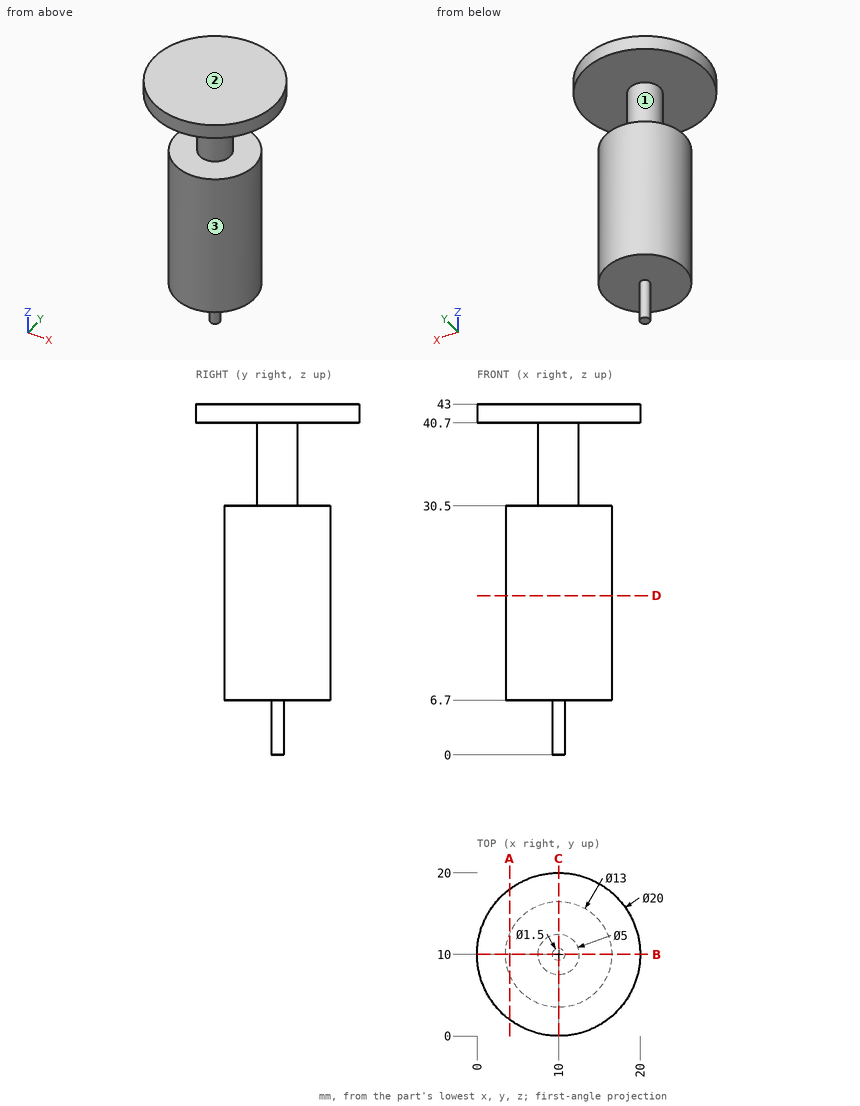
Input: dimensioned drawing with shaded views. Units: mm. Origin: part minimum x, y, z. A direction names the side the tool comes from. Give positions to 0.01 mm unless a question says otherwise; leave off trailing zeros. Loops run counter-clockwise (first coordinate to the right, second up) from the corner with the lowest first, then second, coordinate; pieces in that order, holes last. Notation, with made-up numbers: (31, 58.25) -> (55, 58.25) arc R23 cw to (55, 85.25) -> close; hole circle Ø9 at (-32, 10.5). An arc over 180 degrees is marked (long way). Use a Markdown table: item, result.
Q1. Ray query, probe 1 along Z at (x, y) = (5.5, 5.5); probe 2 along Z at (x, y) = (12, 17.75); probe 3 along X at (y, z) = (5.5, 41). Return the intervals inside material, ascending. Write a range as from..to.
Entries:
| item | result |
|---|---|
| probe 1 | z = 6.7..30.5, 40.7..43 |
| probe 2 | z = 40.7..43 |
| probe 3 | x = 1.07..18.93 |
Q2. Access query for the marked faces 1, 2 and 3. Directions: +Z, -Z, +X, -X, +Y, -Y. A direction counts if a zero-diameter tool reaches every point of the face in a straight line with its end or side. Return the directions, or none.
Entries:
| item | result |
|---|---|
| face 1 | none |
| face 2 | +Z, +X, -X, +Y, -Y |
| face 3 | -Z |
Q3. Section query B-B, the plane y = 10. Return the cut outline in (x, z).
Entries:
| item | result |
|---|---|
| outline | (0, 40.7) -> (7.5, 40.7) -> (7.5, 30.5) -> (3.5, 30.5) -> (3.5, 6.7) -> (9.25, 6.7) -> (9.25, 0) -> (10.75, 0) -> (10.75, 6.7) -> (16.5, 6.7) -> (16.5, 30.5) -> (12.5, 30.5) -> (12.5, 40.7) -> (20, 40.7) -> (20, 43) -> (0, 43) -> close |
Q4. Section query D-D, the plane z = 19.5. Return the cut outline in (x, y).
Entries:
| item | result |
|---|---|
| outline | circle Ø13 at (10, 10) |
Q5. Section query A-A, the plane x = 4. Return the cut outline in (y, z), plus the area to 3 significant figures.
Entries:
| item | result |
|---|---|
| outline | (2, 40.7) -> (18, 40.7) -> (18, 43) -> (2, 43) -> close; (7.5, 6.7) -> (12.5, 6.7) -> (12.5, 30.5) -> (7.5, 30.5) -> close |
| area | 156 mm² |
Q6. First-contact query: P1, Ø1, axis at x = 11, z = 24.5, coming from the -Y side; P2, Ø2, axis at x = 12.5, y = 7, coming from the -Z side; P3, Ø2, axis at x = 13, z = 21.5, coming from the +Y side (1 decimal). Flat tips, straight axial feed; report the tip coordinate or a pass-through.
Entries:
| item | result |
|---|---|
| P1 | stops at y = 3.52 |
| P2 | stops at z = 6.7 |
| P3 | stops at y = 16.2 |
